from build123d import *

# Parameters (mm, degrees)
BASE_FLANGE1_DEPTH           = 1.5875
EDGE_FLANGE1_STRIP_W         = 9.5504
EDGE_FLANGE1_STRIP_H         = 1.5875
EDGE_FLANGE1_STRIP_CUT_DEPTH = 304.8
EDGE_FLANGE1_DEPTH           = 304.8
CUT_EXTRUDE1_DEPTH           = 342.722050796
CUT_EXTRUDE1_DEPTH_BACK      = 342.722050796
F_6_CLEARANCE_HOLE1_D        = 3.7973
F_6_CLEARANCE_HOLE2_D        = 3.7973


# Sheet-metal steps are written as plain solids
with BuildPart() as part:
    # Sketch1 → Base-Flange1 (new body)
    with BuildSketch(Plane(origin=(0, 0, 0), x_dir=(1, 0, 0), z_dir=(0, 1, 0))):
        Polygon((0, 304.8), (76.2, 304.8), (152.4, 0), (0, 0), align=None)
    extrude(amount=-BASE_FLANGE1_DEPTH)

    # Edge-Flange1 strip (across the edge) → Edge-Flange1 strip cut (cut)
    with BuildSketch(Plane(origin=(0, -1.5875, 0), x_dir=(1, 0, 0), z_dir=(0, 0, -1))):
        with Locations((-1.5875, -0.79375)):
            Rectangle(EDGE_FLANGE1_STRIP_W, EDGE_FLANGE1_STRIP_H)
    extrude(amount=EDGE_FLANGE1_STRIP_CUT_DEPTH, mode=Mode.SUBTRACT)

    # Edge-Flange1 section (across the edge) → Edge-Flange1 (add)
    with BuildSketch(Plane(origin=(0, -1.5875, 0), x_dir=(1, 0, 0), z_dir=(0, 0, -1))):
        with BuildLine():
            Line((0, 1.6002), (0, 25.4))
            Line((0, 25.4), (1.5875, 25.4))
            Line((1.5875, 25.4), (1.5875, 1.6002))
            ThreePointArc((1.5875, 1.6002), (2.056187729, 0.468687729), (3.1877, 0))
            Line((3.1877, 0), (3.1877, -1.5875))
            ThreePointArc((3.1877, -1.5875), (0.933655714, -0.653844286), (0, 1.6002))
        make_face()
    extrude(amount=EDGE_FLANGE1_DEPTH)

    # Sketch9 → Cut-Extrude1 (cut, two sides: drawn at the far end of the back side and taken through both)
    with BuildSketch(Plane(origin=(0, -1.5875, 0), x_dir=(-1, 0, 0), z_dir=(0, -1, 0)).offset(-CUT_EXTRUDE1_DEPTH_BACK)):
        Polygon((-67.85590566, 967.941443334), (-67.85590566, 304.8), (-67.85590566, 261.227267277), (-68.183918061, 258.867768839), (-116.937952517, 113.626422367), (-117.240761897, 112.724334108), (-117.240761897, 0), (-117.240761897, -663.141443334), (-1442.916152839, -623.003514641), (-1393.531296603, 1008.079372028), align=None)
    extrude(amount=CUT_EXTRUDE1_DEPTH + CUT_EXTRUDE1_DEPTH_BACK, mode=Mode.SUBTRACT)

    # #6 Clearance Hole1 (through all)
    with Locations(Plane(origin=(0, 0, 0), x_dir=(1, 0, 0), z_dir=(0, 1, 0))):
        with Locations((58.564398425, 260.349999742)):
            Hole(F_6_CLEARANCE_HOLE1_D / 2)

    # #6 Clearance Hole2 (through all)
    with Locations(Plane(origin=(0, 0, 0), x_dir=(1, 0, 0), z_dir=(0, 1, 0))):
        with Locations((107.989583034, 31.750001764), (107.989583034, 63.500001764)):
            Hole(F_6_CLEARANCE_HOLE2_D / 2)


solid = part.part
Verification items for the finished model (mm, model axes). A direction names the side the tool comes from. Round coordinates to 2 decimals unless told otherwise and drop trailing zeros. Loops run counter-clockwise (first coordinate to the right, second up) from the corner with the lowest first, then second, coordinate; pieces in that order, holes last. Notation, with made-up numbers: (-36.75, 32) - (-30.75, 32) arc R23 ccw to (-30.75, 53) - close; hole circle Ø4 at (73, 30.5). An arc over 180 degrees is marked (long way). Use a Markdown table: item, result. Add a question column.
1. Access from +Z, -Z, +X, -X, +Y, -Y to the whole of each face (thin tool, end or side, straight path). Record for faces 1 (the face through (0, -15, -150)), 2 (the face through (48, -1.588, -121)).
2. Section check D-D, the plane z = -71.5. Record the boundary of the cut face in (x, y).
3. Section check C-C, the plane y = -11.5. Record the boundary of the cut face in (x, z).
4. Gauge pin test, flat ends, axial feed: pin 1 (0.8 mm diameter, centred on y = -1, z = -281, fed in from +X); pin 2 (2 mm diameter, centred on y = -8, z = -118.5, fed in from +X); pin 3 (3 mm diameter, centred on x = 96.5, z = -145, fed in from -Y). Record the tip position at first contact, or that the pin passes through.
5. Thickness scan on probe 1 along X at (y, z) = (-19.5, -197.5); probe 2 along Y at (x, z) = (80, -209.5). Record the ranges inside material, lowest first. Write a range as [from, to].
6. Section check A-A, the plane z = -269. Record the boundary of the cut face in (x, y).
7. Section check B-B, the plane x = 46. Record the boundary of the cut face in (y, z), plus the area to 3 significant figures.
Checks:
| question | item | result |
|---|---|---|
| 1 | face 1 | +Z, -Z, -X, +Y, -Y |
| 1 | face 2 | +Z, -Z, +X, -Y |
| 2 | outline | (0, -26.99) - (1.59, -26.99) - (1.59, -3.19) arc R1.6 cw to (3.19, -1.59) - (117.24, -1.59) - (117.24, 0) - (3.19, 0) arc R3.19 ccw to (0, -3.19) - close |
| 3 | outline | (0, -304.8) - (1.59, -304.8) - (1.59, 0) - (0, 0) - close |
| 4 | pin 1 | stops at x = 67.86 |
| 4 | pin 2 | stops at x = 1.59 |
| 4 | pin 3 | stops at y = -1.59 |
| 5 | probe 1 | x = [0, 1.59] |
| 5 | probe 2 | y = [-1.59, 0] |
| 6 | outline | (0, -26.99) - (1.59, -26.99) - (1.59, -3.19) arc R1.6 cw to (3.19, -1.59) - (67.86, -1.59) - (67.86, 0) - (3.19, 0) arc R3.19 ccw to (0, -3.19) - close |
| 7 | outline | (-1.59, -304.8) - (0, -304.8) - (0, 0) - (-1.59, 0) - close |
| 7 | area | 484 mm^2 |
